from build123d import *

# Parameters (mm, degrees)
PAD_DEPTH    = 13.5
SKETCH001_R  = 2.2
POCKET_DEPTH = 12.001
FILLET001_R  = 0.5


with BuildPart() as part:
    # Sketch → Pad (new body, symmetric)
    with BuildSketch(Plane.XY):
        Polygon((-10, 10), (11, 10), (11, 5.25), (1, 7.75), (1, -7.75), (11, -5.25), (11, -10), (-7, -10), (-7, -4), (-10, -4), (-10, -3), (-11, -3), (-11, 3), (-10, 3), align=None)
    extrude(amount=PAD_DEPTH, both=True)

    # Sketch001 (on Face6 of Pad) → Pocket (cut, through all)
    with BuildSketch(Plane.YZ.offset(1)):
        Circle(SKETCH001_R)
    extrude(amount=-POCKET_DEPTH, mode=Mode.SUBTRACT)

    # Fillet001
    fillet001_edges = [part.edges().sort_by_distance(p)[0] for p in [
        (1, 7.75, 0),
        (1, -7.75, 0),
        (11, -5.25, 0),
        (11, 5.25, 0),
    ]]
    fillet(fillet001_edges, radius=FILLET001_R)


solid = part.part
Build history of the part. All positions in model axes, mm. A direction names the side the tool comes from. Coordinates: 2 decimals unless noted, no trailing zeros. Order: outer loops, then holes, each group sorted by start corner. A loop starts at its lowest first (then second) coordinate and runs counter-clockwise, first axis right, second up. Notation, with made-up numbers: (-17.75, 22.25) - (39.25, 22.25) arc R21 cw to (39.25, 30.25) - close; hole circle Ø8 at (-5, 56). An arc over 180 degrees is marked (long way). Write each question's results on one line, items separated by ' | '. Start each with the question number.
Item 1: Band-saw the part on C-C on x = 8.5. Write the cut outline in (y, z) (3 decimals).
Item 2: Band-saw the part on D-D on x = -1.25. Write the cut outline in (y, z).
Item 3: Flat gauge pins, fed straight in: pin 1 (0.9 mm diameter, centred on x = -8, z = 2, fed in from -Y); pin 2 (3.5 mm diameter, centred on y = 0, z = 0, fed in from -X); pin 3 (0.5 mm diameter, centred on y = -3.5, z = -1.5, fed in from -X); pin 4 (1.5 mm diameter, centred on y = 4.5, z = -6.5, fed in from +X). Where does each tip first touch, or does it go through?
Item 4: Band-saw the part on B-B on z = 0. Write the cut outline in (x, y), and give its area (3 significant figures).
Item 5: Mould opens along X. For faces 5 (the face through (11, -8, 0)), 6 (the face through (2, -10, 0)), 7 (the face through (6.061, 6.485, 0.189)) say: released by +X, released by -X, zero draft, split by the parting line, or undercut.
Item 6: Wall check: probe 1 along Z at (x, y) = (-7.5, 0); probe 2 along X at (y, z) = (0.5, -3); probe 3 along X at (y, z) = (8, -8.5). Give the ranges that are in metal, low to high. Write a range as [from, to].
Item 7: Band-saw the part on A-A on y = 6.75. Write the cut outline in (x, z), and give its area (3 significant figures).
Item 8: Tool access for faces 1 (the face through (1, 0, 3)), 2 (the face through (-8, -4, 0)), 3 (the face through (0, 10, 0)), 4 (the face through (-10.5, 3, 0.2)): list every direction of +Z, -Z, +X, -X, +Y, -Y with a clear straight run to the whole face (end or side of a thin tool).
Numbers:
1) outline: (-10, -13.5) - (-5.875, -13.5) - (-5.875, 13.5) - (-10, 13.5) - close; (5.875, -13.5) - (10, -13.5) - (10, 13.5) - (5.875, 13.5) - close
2) outline: (-10, -13.5) - (10, -13.5) - (10, 13.5) - (-10, 13.5) - close; hole circle Ø4.4 at (0, 0)
3) pin 1: y = -4 | pin 2: through | pin 3: x = -10 | pin 4: x = 1
4) outline: (-11, -3) - (-10, -3) - (-10, -4) - (-7, -4) - (-7, -10) - (11, -10) - (11, -5.89) arc R0.5 ccw to (10.38, -5.41) - (1.62, -7.59) arc R0.5 cw to (1, -7.11) - (1, -2.2) - (-11, -2.2) - close; (-11, 2.2) - (1, 2.2) - (1, 7.11) arc R0.5 cw to (1.62, 7.59) - (10.38, 5.41) arc R0.5 ccw to (11, 5.89) - (11, 10) - (-10, 10) - (-10, 3) - (-11, 3) - close | area: 225 mm^2
5) face 5: released by +X | face 6: zero draft | face 7: undercut
6) probe 1: [-13.5, -2.2], [2.2, 13.5] | probe 2: [-11, 1] | probe 3: [-10, 11]
7) outline: (-10, -13.5) - (1, -13.5) - (1, 13.5) - (-10, 13.5) - close; (5, -13.5) - (11, -13.5) - (11, 13.5) - (5, 13.5) - close | area: 459 mm^2
8) face 1: +Z, -Z | face 2: +Z, -Z, -X, -Y | face 3: +Z, -Z, +X, -X, +Y | face 4: +Z, -Z, -X, +Y
